The model under review builds one solid part; all positions refer to its coordinate system, in mm. A direction names the side the tool comes from. Round coordinates to 2 decimals unless told otherwise and drop trailing zeros. Write each loop counter-clockwise with the first axis right and the second up, starting at its lowest first coordinate (ties: lowest second). Pieces come first, ordered by that corner, then holes. Notation, with made-up numbers: (84, 35) - (143, 35) arc R36 ccw to (143, 74) - close; hole circle Ø3 at (-12.5, -18.75). An arc over 180 degrees is marked (long way). Use one line per item in the form item = value.
from build123d import *

# Parameters (mm, degrees)
SKETCH1_W           = 230
SKETCH1_H           = 230
BOSS_EXTRUDE1_DEPTH = 20
SKETCH2_R           = 3.4
CUT_EXTRUDE1_DEPTH  = 21
SKETCH3_W           = 230
SKETCH3_H           = 20
BOSS_EXTRUDE2_DEPTH = 100


with BuildPart() as part:
    # Sketch1 → Boss-Extrude1 (new body)
    with BuildSketch(Plane.ZY.offset(23545.4736246)):
        with Locations((40171.936259601, 5861.690204874)):
            Rectangle(SKETCH1_W, SKETCH1_H)
    extrude(amount=BOSS_EXTRUDE1_DEPTH)

    # Sketch2 → Cut-Extrude1 (cut, through all)
    with BuildSketch(Plane.ZY.offset(23565.4736246)):
        with Locations((40187.941310235, 5920.121662379)):
            Circle(SKETCH2_R)
        with Locations((40230.367717106, 5877.695255508)):
            Circle(SKETCH2_R)
        with Locations((40145.514903364, 5877.695255508)):
            Circle(SKETCH2_R)
    extrude(amount=-CUT_EXTRUDE1_DEPTH, mode=Mode.SUBTRACT)

    # Sketch3 → Boss-Extrude2 (add)
    with BuildSketch(Plane.ZY.offset(23565.4736246)):
        with Locations((40171.936259601, 5756.690204874)):
            Rectangle(SKETCH3_W, SKETCH3_H)
    extrude(amount=BOSS_EXTRUDE2_DEPTH)


solid = part.part
(1) Add section D-D on y = 5854. Write out the cut boundary in (x, z).
Geometry results:
outline = (-23565.47, 40056.94) - (-23545.47, 40056.94) - (-23545.47, 40286.94) - (-23565.47, 40286.94) - close
(2) To check wall thickness, follow L1, parallel to X at y = 5929, z = 40166; L2, parallel to Y at x = -23602.5, z = 40121. State the ranges of each line that lie inside material, in increasing order.
Geometry results:
L1 = -23565.47 to -23545.47
L2 = 5746.69 to 5766.69
(3) Add section B-B on x = -23572. Write out the cut boundary in (y, z), then the cut area to 3 significant figures.
Geometry results:
outline = (5746.69, 40056.94) - (5766.69, 40056.94) - (5766.69, 40286.94) - (5746.69, 40286.94) - close
area = 4,600 mm2
(4) Insertion check: P1, Ø3, axis at y = 5871.5, z = 40207, coming from the -X side; P2, Ø5, axis at x = -23635, z = 40141.5, coming from the +Y side. Each pin has a flat end and moves straight along its axis. Give the tip position at first contact, or say it passes through.
Geometry results:
P1 = -23565.47
P2 = 5766.69
(5) Add section C-C on z = 40230.5. Write out the cut boundary in (x, y), then the cut area to 3 significant figures.
Geometry results:
outline = (-23665.47, 5746.69) - (-23545.47, 5746.69) - (-23545.47, 5874.3) - (-23565.47, 5874.3) - (-23565.47, 5766.69) - (-23665.47, 5766.69) - close; (-23565.47, 5881.09) - (-23545.47, 5881.09) - (-23545.47, 5976.69) - (-23565.47, 5976.69) - close
area = 6,460 mm2
(6) The part is to be moulded in two halves that separate along Y. For faces 3 (the flat face through (-23545.474, 5863, 40170)), 4 (the flat face through (-23555, 5976.69, 40170)), 5 (the cylindrical face through (-23555.614, 5921.143, 40191.184)), say which applies: +Y half, -Y half, draft (parallel to the pull), parting line (faces both ways), or undercut.
Geometry results:
face_3 = draft
face_4 = +Y half
face_5 = undercut
(7) Machinability: for faces 1 (the flat face through (-23615, 5766.69, 40170)), 2 (the cylindrical face through (-23555.614, 5878.717, 40148.758)), which of the approach directions +Z, -Z, +X, -X, +Y, -Y give a long, thin tool a straight path to every point of the face, cutting with its end or side? Answer none if there is none.
Geometry results:
face_1 = +Z, -Z, -X, +Y
face_2 = +X, -X
(8) Add section A-A on z = 40112. Write out the cut boundary in (x, y), then the cut area to 3 significant figures.
Geometry results:
outline = (-23665.47, 5746.69) - (-23545.47, 5746.69) - (-23545.47, 5976.69) - (-23565.47, 5976.69) - (-23565.47, 5766.69) - (-23665.47, 5766.69) - close
area = 6,600 mm2
